```python
from build123d import *

# Parameters (mm, degrees)
SKETCH1_W           = 70
SKETCH1_H           = 50
BOSS_EXTRUDE1_DEPTH = 1
SKETCH2_R           = 1.4
CUT_EXTRUDE1_DEPTH  = 87.029064856
SKETCH3_W           = 18.365703091
SKETCH3_H           = 7.700561822
SKETCH3_W_2         = 18.038456085
SKETCH3_W_3         = 17.313956014
BOSS_EXTRUDE2_DEPTH = 10
SKETCH4_R           = 2.199397545
SKETCH4_R_2         = 2.613331078
SKETCH4_W           = 6.039158021
SKETCH4_H           = 5.855225109
SKETCH4_W_2         = 4.288386861
SKETCH4_H_2         = 8.320722996
BOSS_EXTRUDE3_DEPTH = 13
SKETCH5_R           = 2.461468561
BOSS_EXTRUDE4_DEPTH = 13


with BuildPart() as part:
    # Sketch1 → Boss-Extrude1 (new body)
    with BuildSketch(Plane(origin=(0, 0, 0), x_dir=(1, 0, 0), z_dir=(0, 1, 0))):
        with Locations((35, 25)):
            Rectangle(SKETCH1_W, SKETCH1_H)
    extrude(amount=BOSS_EXTRUDE1_DEPTH)

    # Sketch2 → Cut-Extrude1 (cut, through all)
    with BuildSketch(Plane(origin=(0, 1, 0), x_dir=(1, 0, 0), z_dir=(0, 1, 0))):
        with Locations(Location((2, 48, 0), (0, 0, 270))):
            Circle(SKETCH2_R)
        with Locations(Location((68, 48, 0), (0, 0, 270))):
            Circle(SKETCH2_R)
        with Locations(Location((68, 2, 0), (0, 0, 270))):
            Circle(SKETCH2_R)
        with Locations(Location((2, 2, 0), (0, 0, 270))):
            Circle(SKETCH2_R)
    extrude(amount=-CUT_EXTRUDE1_DEPTH, mode=Mode.SUBTRACT)

    # Sketch3 → Boss-Extrude2 (add)
    with BuildSketch(Plane(origin=(0, 1, 0), x_dir=(1, 0, 0), z_dir=(0, 1, 0))):
        with Locations((14.447202749, 25.749679834)):
            Rectangle(SKETCH3_W, SKETCH3_H)
        with Locations((34.720477754, 25.749679834)):
            Rectangle(SKETCH3_W_2, SKETCH3_H)
        with Locations((56.000727736, 25.749679834)):
            Rectangle(SKETCH3_W_3, SKETCH3_H)
    extrude(amount=BOSS_EXTRUDE2_DEPTH)

    # Sketch4 → Boss-Extrude3 (add)
    with BuildSketch(Plane(origin=(0, 1, 0), x_dir=(1, 0, 0), z_dir=(0, 1, 0))):
        with Locations(Location((11.812429649, 5.207282589, 0), (0, 0, 90))):
            Circle(SKETCH4_R)
        with Locations(Location((49.177509177, 42.774595264, 0), (0, 0, 90))):
            Circle(SKETCH4_R_2)
        with Locations((48.771261245, 7.170254424)):
            Rectangle(SKETCH4_W, SKETCH4_H)
        with Locations((66.789850866, 14.979105773)):
            Rectangle(SKETCH4_W_2, SKETCH4_H_2)
    extrude(amount=BOSS_EXTRUDE3_DEPTH)

    # Sketch5 → Boss-Extrude4 (add)
    with BuildSketch(Plane(origin=(0, 1, 0), x_dir=(1, 0, 0), z_dir=(0, 1, 0))):
        with Locations(Location((6.367279466, 5.676618651, 0), (0, 0, 90))):
            Circle(SKETCH5_R)
    extrude(amount=BOSS_EXTRUDE4_DEPTH)


solid = part.part
```
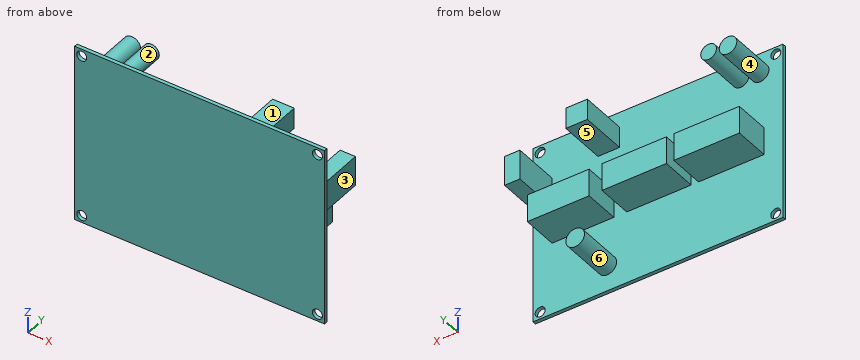
The listing builds one solid part. Answer for the finished solid, in the listing's coordinates (mm). Face numbers are marked on the shaded views. A direction names the side the tool comes from. Give positions to 0.01 mm unless a question says otherwise; leave off trailing zeros. Order: outer loops, then holes, each group sorted by start corner. A loop starts at its lowest first (then second) coordinate and runs counter-clockwise, first axis right, second up. Notation, with made-up numbers: (48, 21.5) - (102, 21.5) arc R24 ccw to (102, 32.5) - close; hole circle Ø5 at (80.25, 52). An arc over 180 degrees is marked (long way). Use one line per item in the form item = value. Start each with the question number.
(1) A cutting plane is placed at D-D, the plane x = 42. Write down the section's boundary in (y, z), then the cut area to 3 significant figures.
(2) Flat-ended cylindrical pins translate along their axes: pin 1 Ø3.5 at (x, y) = (66, 8) entering from -Z; pin 2 Ø8.5 at (x, z) = (54, -26.5) entering from +Y; pin 3 Ø8 at (x, y) = (34.5, 6) entering from +Z. Find the tip coordinate at first contact, or state that the pin passes through.
(3) For the marked faces 1, 2 and 3, determine the directions among +Z, -Z, +X, -X, +Y, -Y from which every point of the face is accessible in a straight line to the end or side of a thin tool.
(4) A cutting plane is placed at A-A, the plane x = 68. Write down the section's boundary in (y, z), then the cut area to 3 significant figures.
(5) The mould has two halves that part along X. Classify the marked faces 4, 5 and 6: released by +X, released by -X, zero draft, split by the parting line, or undercut.
(6) A cutting plane is placed at B-B, the plane y = 12. Write down the section's boundary in (x, z).
(7) A cutting plane is placed at C-C, the plane z = -2. Write down the section's boundary in (x, y).
(8) Consider line 1 (X direction, y = 0.3, z = -48); line 2 (Z direction, x = 68, y = 0.5); line 3 (X direction, y = 7.25, z = -22). Determine where each line is inside the solid, lowest interval first. Write a range as from..to.
Ans:
q1.outline = (0, -50) - (1, -50) - (1, -29.6) - (11, -29.6) - (11, -21.9) - (1, -21.9) - (1, 0) - (0, 0) - close
q1.area = 127 mm^2
q2.pin_1 = -29.6
q2.pin_2 = 11
q2.pin_3 = -21.9
q3.face_1 = +Z, +X, +Y
q3.face_2 = +Y
q3.face_3 = +Z, -Z, +X, +Y
q4.outline = (0, -50) - (1, -50) - (1, -49.4) - (0, -49.4) - close; (0, -46.6) - (1, -46.6) - (1, -19.14) - (14, -19.14) - (14, -10.82) - (1, -10.82) - (1, -3.4) - (0, -3.4) - close; (0, -0.6) - (1, -0.6) - (1, 0) - (0, 0) - close
q4.area = 153 mm^2
q5.face_4 = undercut
q5.face_5 = zero draft
q5.face_6 = split by the parting line
q6.outline = circle Ø4.92 at (6.37, -5.68); circle Ø4.4 at (11.81, -5.21); (45.75, -10.1) - (51.79, -10.1) - (51.79, -4.24) - (45.75, -4.24) - close; circle Ø5.23 at (49.18, -42.77); (64.65, -19.14) - (68.93, -19.14) - (68.93, -10.82) - (64.65, -10.82) - close
q7.outline = (0, 0) - (0.6, 0) - (0.6, 1) - (0, 1) - close; (3.4, 0) - (66.6, 0) - (66.6, 1) - (3.4, 1) - close; (69.4, 0) - (70, 0) - (70, 1) - (69.4, 1) - close
q8.line_1 = 0..0.6, 3.4..66.6, 69.4..70
q8.line_2 = -50..-49.4, -46.6..-3.4, -0.6..0
q8.line_3 = 5.26..23.63, 25.7..43.74, 47.34..64.66
